```python
from build123d import *

# Parameters (mm, degrees)
BOSS_EXTRUDE1_DEPTH     = 33
CUT_EXTRUDE1_DEPTH      = 60
SKETCH3_W               = 125.025821482
SKETCH3_H               = 26
CUT_EXTRUDE2_DEPTH      = 25
CUT_EXTRUDE6_DEPTH      = 98.759359099
CUT_EXTRUDE6_DEPTH_BACK = 98.759359099
SKETCH7_W               = 50
SKETCH7_H               = 26
SKETCH8_W               = 91.898790586
SKETCH8_H               = 33
BOSS_EXTRUDE2_DEPTH     = 3
FILLET1_R               = 3


with BuildPart() as part:
    # Sketch1 → Boss-Extrude1 (new body)
    with BuildSketch(Plane.XY):
        with BuildLine():
            Line((-62.512910741, 10.211947396), (62.512910741, 10.211947396))
            ThreePointArc((62.512910741, 10.211947396), (88.5, 0), (62.512910741, -10.211947396))
            Line((62.512910741, -10.211947396), (-62.512910741, -10.211947396))
            ThreePointArc((-62.512910741, -10.211947396), (-88.5, 0), (-62.512910741, 10.211947396))
        make_face()
    extrude(amount=BOSS_EXTRUDE1_DEPTH)

    # Sketch2 → Cut-Extrude1 (cut)
    with BuildSketch(Plane.XY.offset(43)):
        with BuildLine():
            Line((44.606109659, 2.95), (-44.606109659, 2.95))
            ThreePointArc((-44.606109659, 2.95), (-47.976180371, 0), (-44.606109659, -2.95))
            Line((-44.606109659, -2.95), (44.606109659, -2.95))
            ThreePointArc((44.606109659, -2.95), (48.007891593, 0), (44.606109659, 2.95))
        make_face()
    extrude(amount=-CUT_EXTRUDE1_DEPTH, mode=Mode.SUBTRACT)

    # Sketch3 → Cut-Extrude2 (cut)
    with BuildSketch(Plane(origin=(0, 10.211947396, 0), x_dir=(1, 0, 0), z_dir=(0, 1, 0))):
        with Locations((0, -16.5)):
            Rectangle(SKETCH3_W, SKETCH3_H)
    extrude(amount=-CUT_EXTRUDE2_DEPTH, mode=Mode.SUBTRACT)

    # Sketch7 → Cut-Extrude6 (cut, two sides: drawn at the far end of the back side and taken through both)
    with BuildSketch(Plane(origin=(0, 10.211947396, 0), x_dir=(-1, 0, 0), z_dir=(0, -1, 0)).offset(-CUT_EXTRUDE6_DEPTH_BACK)):
        with Locations((87.512910741, -16.5)):
            Rectangle(SKETCH7_W, SKETCH7_H)
    extrude(amount=CUT_EXTRUDE6_DEPTH + CUT_EXTRUDE6_DEPTH_BACK, mode=Mode.SUBTRACT)

    # Sketch8 → Boss-Extrude2 (add)
    with BuildSketch(Plane(origin=(0, 10.211947396, 0), x_dir=(1, 0, 0), z_dir=(0, 1, 0))):
        with Locations((0, -16.5)):
            Rectangle(SKETCH8_W, SKETCH8_H)
    extrude(amount=BOSS_EXTRUDE2_DEPTH)

    # Fillet1
    fillet1_edges = [part.edges().sort_by_distance(p)[0] for p in [
        (0, 13.211947396, 0),
        (0, 13.211947396, 33),
    ]]
    fillet(fillet1_edges, radius=FILLET1_R)


solid = part.part
```
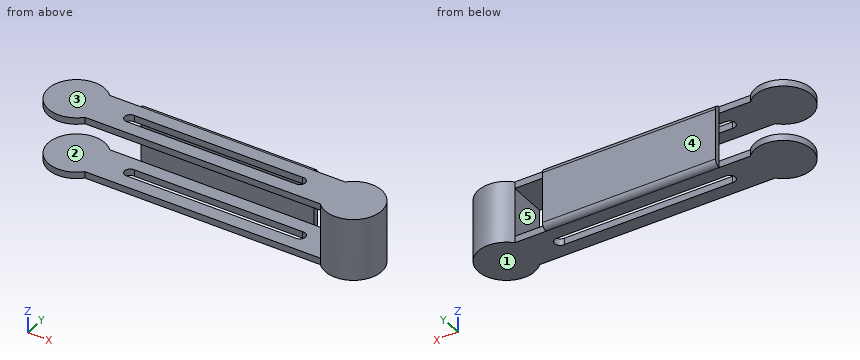
CAD build for the part. Positions are in the model's coordinates, mm. Face numbers are marked on the shaded views. A direction names the side the tool comes from. Give positions to 0.01 mm unless a question says otherwise; leave off trailing zeros. Order: outer loops, then holes, each group sorted by start corner. A loop starts at its lowest first (then second) coordinate and runs counter-clockwise, first axis right, second up. Notation, with made-up numbers: M -38.5,23 L -16.5,23 A24 cw -16.5,43 Z; hole C -32,78 d3. An arc over 180 degrees is marked long. Put each result on its own line as item: value. Start each with the question number.
(1) Flat gauge pins, fed straight in: pin 1 Ø7 at (x, y) = (45.03, 0) entering from -Z; pin 2 Ø1.8 at (x, z) = (54.5, 31) entering from +Y; pin 3 Ø13.5 at (x, z) = (0, 10) entering from +Y; pin 4 Ø3 at (y, z) = (-7.5, 9) entering from +X. Where does each tip first touch, or does it go through?
(2) Mould opens along Z. For the marked faces 3, 4 and 5 say: +Z half, -Z half, draft (parallel to the pull), parting line (faces both ways), or undercut.
(3) Saw through at A-A, the plane x = -73.5. Write the cut outline in (y, z).
(4) Saw through at D-D, the plane y = 6. Write the cut outline in (x, z).
(5) Drill centre lines: line 1 along Z through (x, y) = (-59, 8); line 2 along X through (y, z) = (10.5, 8); line 3 along Y through (x, z) = (-45, 2). Where is each one in solid material? Low to high.
(6) Which spindle directions (+Z, -Z, +X, -X, +Y, -Y) get a long thin tool onto all of the face, cutting with end or side? Do the marked faces 1 and 2. Say none if no direction does.
(7) Saw through at C-C, the plane x = -4. Write the cut outline in (y, z), then the cut area to 3 significant figures.
(8) Saw through at B-B, the plane z = 22. Write the cut outline in (x, y), then the cut area to 3 significant figures.
Check result:
1. pin 1: stops at z = 0
1. pin 2: stops at y = 10.21
1. pin 3: stops at y = 13.21
1. pin 4: stops at x = 87.25
2. face 3: +Z half
2. face 4: draft
2. face 5: undercut
3. outline: M -15,0 L 15,0 L 15,3.5 L -15,3.5 Z; M -15,29.5 L 15,29.5 L 15,33 L -15,33 Z
4. outline: M -87.25,0 L 87.25,0 L 87.25,33 L -87.25,33 L -87.25,29.5 L 62.51,29.5 L 62.51,3.5 L -87.25,3.5 Z
5. line 1: z = 0 to 3.5, 29.5 to 33
5. line 2: x = -45.95 to 45.95, 62.79 to 84.21
5. line 3: y = -10.21 to -2.98, 2.98 to 13.04
6. face 1: -Z, +X, -X, +Y, -Y
6. face 2: -X, -Y
7. outline: M -10.21,0 L -2.95,0 L -2.95,3.5 L -10.21,3.5 Z; M -10.21,29.5 L -2.95,29.5 L -2.95,33 L -10.21,33 Z; M 2.95,0 L 10.21,0 A3 ccw 13.21,3 L 13.21,30 A3 ccw 10.21,33 L 2.95,33 L 2.95,29.5 L 10.21,29.5 L 10.21,3.5 L 2.95,3.5 Z
7. area: 197 mm2
8. outline: M -45.95,10.21 L 45.95,10.21 L 45.95,13.21 L -45.95,13.21 Z; M 62.51,-10.21 A15 ccw long 62.51,10.21 Z
8. area: 926 mm2
